Design review of the part built by this model. Coordinates are the model's own, in mm. Coordinates: 2 decimals unless noted, no trailing zeros. Loops run counter-clockwise (first coordinate to the right, second up) from the corner with the lowest first, then second, coordinate; pieces in that order, holes last. Notation, with made-up numbers: M 61,-13 L 69,-13 A21 ccw 69,1 Z; hole C -37,-3 d7. An arc over 180 degrees is marked long. Answer as a JSON object with one key per item and string values. Group by question number.
1. Insertion check: pin 1 (16 mm diameter, centred on x = -110, z = 15, fed in from +Y). The pin has a flat end and moves straight along its axis. Give the tip position at first contact, or say it passes through.
2. Consider section B-B (z = 15). State the section outline as (x, y) points, then the cut area to 3 significant figures.
3. Consider section C-C (y = 4.45). State the section outline as (x, z) points.
4. To check wall thickness, follow probe 1 along X at (y, z) = (1.5, 15); probe 2 along Z at (x, y) = (-110, 3.5). State the ranges of each line that lie inside material, in increasing order.
5. Consider section A-A (x = -110). State the section outline as (y, z) points, then the cut area to 3 significant figures.
from build123d import *

# Parameters (mm, degrees)
SKETCH1_W               = 260
SKETCH1_H               = 60
BOSS_EXTRUDE1_DEPTH     = 6
CUT_EXTRUDE1_DEPTH      = 134.551488198
CUT_EXTRUDE1_DEPTH_BACK = 134.551488198
SKETCH2_R               = 7


with BuildPart() as part:
    # Sketch1 → Boss-Extrude1 (new body)
    with BuildSketch(Plane(origin=(0, 0, 0), x_dir=(1, 0, 0), z_dir=(0, 1, 0))):
        Rectangle(SKETCH1_W, SKETCH1_H)
    extrude(amount=BOSS_EXTRUDE1_DEPTH)

    # Sketch2 → Cut-Extrude1 (cut, two sides: drawn at the far end of the back side and taken through both)
    with BuildSketch(Plane(origin=(0, 6, 0), x_dir=(1, 0, 0), z_dir=(0, 1, 0)).offset(-CUT_EXTRUDE1_DEPTH_BACK)):
        with Locations(Location((110, -15, 0), (0, 0, 270))):
            Circle(SKETCH2_R)
        with Locations(Location((-110, -15, 0), (0, 0, 270))):
            Circle(SKETCH2_R)
    extrude(amount=CUT_EXTRUDE1_DEPTH + CUT_EXTRUDE1_DEPTH_BACK, mode=Mode.SUBTRACT)


solid = part.part
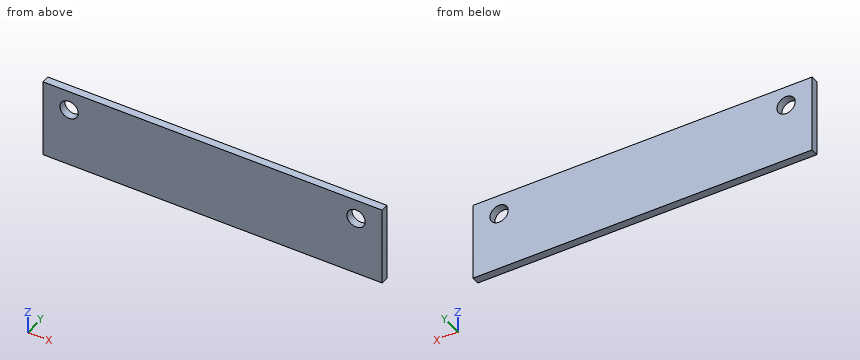
Findings below:
{
 "1": {"pin 1": "stops at y = 6"},
 "2": {"outline": "M -130,0 L -117,0 L -117,6 L -130,6 Z; M -103,0 L 103,0 L 103,6 L -103,6 Z; M 117,0 L 130,0 L 130,6 L 117,6 Z", "area": "1,390 mm^2"},
 "3": {"outline": "M -130,-30 L 130,-30 L 130,30 L -130,30 Z; hole C -110,15 d14; hole C 110,15 d14"},
 "4": {"probe 1": "x = -130 to -117, -103 to 103, 117 to 130", "probe 2": "z = -30 to 8, 22 to 30"},
 "5": {"outline": "M 0,-30 L 6,-30 L 6,8 L 0,8 Z; M 0,22 L 6,22 L 6,30 L 0,30 Z", "area": "276 mm^2"}
}
